Source: CAD feature listing. Evaluate the final solid. Frame: model axes, mm. A direction names the side the tool comes from. Give positions to 0.01 mm unless a question says otherwise; leave off trailing zeros. Write each loop counter-clockwise with the first axis right and the second up, starting at its lowest first coordinate (ties: lowest second). Pieces come first, ordered by that corner, then holes. Notation, with made-up numbers: M 47,20.5 L 87,20.5 A27 cw 87,58.5 Z; hole C 60.5,-10 d11. An arc over 180 degrees is marked long. Answer as a JSON object with one key per item and string values. Group by question number.
```python
from build123d import *

# Parameters (mm, degrees)
F0_W     = 10
F0_H     = 10
F1_DEPTH = 20
F2_R     = 5
F2_R_2   = 2.5
F3_DEPTH = 86.8
F4_DEPTH = 10
F5_R     = 5
F5_R_2   = 2.5
F6_DEPTH = 102.9
F7_DEPTH = 10


with BuildPart() as f1:
    # F0 (on Top) → F1 (new body)
    with BuildSketch(Plane.XY):
        Polygon((-45.7201178421, 45.7201178421), (-55.7201178421, 45.7201178421), (-55.7201178421, -44.2798821579), (-45.7201178421, -44.2798821579), (-45.7201178421, -32.9700666645), (-45.7201178421, -27.9700666645), (-45.7201178421, -5), (-45.7201178421, 0), (-45.7201178421, 24.1741651532), (-45.7201178421, 29.1741651532), align=None)
        with Locations((-50.7201178421, 50.7201178421)):
            Rectangle(F0_W, F0_H)
        Polygon((44.2798821579, 55.7201178421), (-45.7201178421, 55.7201178421), (-45.7201178421, 45.7201178421), (-29.1741651532, 45.7201178421), (-24.1741651532, 45.7201178421), (0, 45.7201178421), (5, 45.7201178421), (27.9700666645, 45.7201178421), (32.9700666645, 45.7201178421), (44.2798821579, 45.7201178421), align=None)
        Polygon((-29.1741651532, 45.7201178421), (-45.7201178421, 29.1741651532), (-45.7201178421, 24.1741651532), (-24.1741651532, 45.7201178421), align=None)
        Polygon((0, 45.7201178421), (-45.7201178421, 0), (-45.7201178421, -5), (5, 45.7201178421), align=None)
        Polygon((-45.7201178421, -32.9700666645), (32.9700666645, 45.7201178421), (27.9700666645, 45.7201178421), (-45.7201178421, -27.9700666645), align=None)
    extrude(amount=F1_DEPTH)

    # F2 (on face) → F3 (cut)
    with BuildSketch(Plane(origin=(-55.7201178421, 0, 0), x_dir=(0, -1, 0), z_dir=(-1, 0, 0))):
        with Locations((9.2798821579, 10)):
            Circle(F2_R)
        with Locations((9.2798821579, 10)):
            Circle(F2_R_2, mode=Mode.SUBTRACT)
        with Locations((-20.7201178421, 10)):
            Circle(F2_R)
        with Locations((-20.7201178421, 10)):
            Circle(F2_R_2, mode=Mode.SUBTRACT)
        with Locations((9.2798821579, 10)):
            Circle(F2_R_2)
        with Locations((-20.7201178421, 10)):
            Circle(F2_R_2)
    extrude(amount=-F3_DEPTH, mode=Mode.SUBTRACT)

    # F2 (on face) → F4 (join)
    with BuildSketch(Plane(origin=(-55.7201178421, 0, 0), x_dir=(0, -1, 0), z_dir=(-1, 0, 0))):
        with Locations((-20.7201178421, 10)):
            Circle(F2_R)
        with Locations((-20.7201178421, 10)):
            Circle(F2_R_2, mode=Mode.SUBTRACT)
        with Locations((9.2798821579, 10)):
            Circle(F2_R)
        with Locations((9.2798821579, 10)):
            Circle(F2_R_2, mode=Mode.SUBTRACT)
    extrude(amount=-F4_DEPTH)

    # F5 (on face) → F6 (cut)
    with BuildSketch(Plane(origin=(0, 55.7201178421, 0), x_dir=(-1, 0, 0), z_dir=(0, 1, 0))):
        with Locations((20.7201178421, 10)):
            Circle(F5_R)
        with Locations((20.7201178421, 10)):
            Circle(F5_R_2, mode=Mode.SUBTRACT)
        with Locations((-9.2798821579, 10)):
            Circle(F5_R)
        with Locations((-9.2798821579, 10)):
            Circle(F5_R_2, mode=Mode.SUBTRACT)
        with Locations((20.7201178421, 10)):
            Circle(F5_R_2)
        with Locations((-9.2798821579, 10)):
            Circle(F5_R_2)
    extrude(amount=-F6_DEPTH, mode=Mode.SUBTRACT)

    # F5 (on face) → F7 (join)
    with BuildSketch(Plane(origin=(0, 55.7201178421, 0), x_dir=(-1, 0, 0), z_dir=(0, 1, 0))):
        with Locations((-9.2798821579, 10)):
            Circle(F5_R)
        with Locations((-9.2798821579, 10)):
            Circle(F5_R_2, mode=Mode.SUBTRACT)
        with Locations((20.7201178421, 10)):
            Circle(F5_R)
        with Locations((20.7201178421, 10)):
            Circle(F5_R_2, mode=Mode.SUBTRACT)
    extrude(amount=-F7_DEPTH)


solid = f1.part
```
(1) Contact query for flat-ended pins moving along their axis: pin 1 Ø12 at (y, z) = (27, 5.5) entering from +X; pin 2 Ø8.5 at (x, z) = (-40.5, 7) entering from -Y; pin 3 Ø10 at (x, z) = (-12, 8.5) entering from -Y. Output: stop coordinate, or through.
(2) Ray query, L1, parallel to Y at x = -3, z = 18; L2, parallel to X at y = 9, z = 17.75; L3, parallel to Y at x = -28, z = 7. Return the intervals inside material, ascending. Write a range as [from, to].
(3) Pull-direction query (X, two-part tool) for faces 1 (the flat face through (44.28, 51, 10)), 2 (the flat face through (-5, 55.72, 10)), 3 (the cylindrical face through (-23.03, 50.79, 9.04)), 4 (the flat face through (-38, 45.72, 10)); classes: pulls with the +X half, pulls with the -X half, needs draft (parallel to the pull), parting line crosses it, or undercut.
(4) Section C-C, the plane x = 23.5. Return loops of the section in (y, z), plus the area to 3 significant figures.
(5) Access query for faces 5 (the cylindrical face through (2.039, 15.723, 9.842)), 6 (the flat face through (-22.54, 23.18, 3.19)), 7 (the cylindrical face through (-15.722, 26.584, 10.141)), 8 (the cylindrical face through (11.264, 50.79, 8.479)). Directions: +Z, -Z, +X, -X, +Y, -Y. A direction counts if a zero-diameter tool reaches every point of the face in a straight line with its end or side. Return the directions, or none.
(6) Section D-D, the plane z = 10. State how many separate pieces and enclosed holes the cut face has, plus the area to 3 significant figures.
(7) Section B-B, the plane z = 3.75. Return loops of the section in (x, y), plus the area to 3 significant figures.
(8) Section A-A, the plane y = 5. Return loops of the section in (x, z).
Reported:
{
 "1": {"pin 1": "stops at x = 20.25", "pin 2": "stops at y = -32", "pin 3": "stops at y = -4"},
 "2": {"L1": "y = [9.75, 14.75], [37.72, 42.72], [45.72, 55.72]", "L2": "x = [-55.72, -45.72], [-36.72, -31.72], [-8.75, -3.75]", "L3": "y = [-15.25, -13.28], [12.72, 16.72], [41.89, 55.72]"},
 "3": {"face 1": "pulls with the +X half", "face 2": "needs draft", "face 3": "undercut", "face 4": "undercut"},
 "4": {"outline": "M 36.25,0 L 41.25,0 L 41.25,20 L 36.25,20 Z; M 45.72,0 L 55.72,0 L 55.72,20 L 45.72,20 Z", "area": "300 mm2"},
 "5": {"face 5": "+X", "face 6": "+Z, -Z", "face 7": "-Y", "face 8": "+Y, -Y"},
 "6": {"separate pieces": "6", "enclosed holes": "1", "area": "2,220 mm2"},
 "7": {"outline": "M -55.72,-44.28 L -45.72,-44.28 L -45.72,-32.97 L 32.97,45.72 L 44.28,45.72 L 44.28,55.72 L -55.72,55.72 Z; hole M -45.72,-27.97 L 27.97,45.72 L 5,45.72 L -45.72,-5 Z; hole M -45.72,0 L 0,45.72 L -24.17,45.72 L -45.72,24.17 Z; hole M -45.72,29.17 L -29.17,45.72 L -45.72,45.72 Z", "area": "2,620 mm2"},
 "8": {"outline": "M -55.72,0 L -45.72,0 L -45.72,20 L -55.72,20 Z; M -40.72,0 L -35.72,0 L -35.72,20 L -40.72,20 Z; M -12.75,0 L -7.75,0 L -7.75,20 L -12.75,20 Z"}
}
